from build123d import *

# Parameters (mm, degrees)
ESQUISSE1_R             = 4
BOSS_EXTRU_1_DEPTH      = 35
ESQUISSE2_R             = 3
ENL_V_MAT_EXTRU_1_DEPTH = 13
BOSS_EXTRU_2_START      = 10
BOSS_EXTRU_2_DEPTH      = 10
ESQUISSE5_R             = 10
ESQUISSE5_R_2           = 4
BOSS_EXTRU_3_DEPTH      = 7


with BuildPart() as part:
    # Esquisse1 → Boss.-Extru.1 (new body)
    with BuildSketch(Plane(origin=(0, 0, 0), x_dir=(1, 0, 0), z_dir=(0, 1, 0))):
        with Locations(Location((0, 0, 0), (0, 0, 270))):
            Circle(ESQUISSE1_R)
    extrude(amount=-BOSS_EXTRU_1_DEPTH)

    # Esquisse2 → Enlèv. mat.-Extru.1 (cut)
    with BuildSketch(Plane(origin=(0, 0, 0), x_dir=(1, 0, 0), z_dir=(0, 1, 0))):
        with Locations(Location((0, 0, 0), (0, 0, 270))):
            Circle(ESQUISSE2_R)
    extrude(amount=-ENL_V_MAT_EXTRU_1_DEPTH, mode=Mode.SUBTRACT)

    # Esquisse4 → Boss.-Extru.2 (add)
    with BuildSketch(Plane(origin=(0, -13, 0), x_dir=(1, 0, 0), z_dir=(0, 1, 0)).offset(BOSS_EXTRU_2_START)):
        with BuildLine():
            Line((-2.41, -1.786588929), (-2.41, 0))
            Line((-2.41, 0), (-2.41, 1.786588929))
            ThreePointArc((-2.41, 1.786588929), (-3, 0), (-2.41, -1.786588929))
        make_face()
    extrude(amount=-BOSS_EXTRU_2_DEPTH)

    # Esquisse5 → Boss.-Extru.3 (add)
    with BuildSketch(Plane(origin=(0, 0, 0), x_dir=(1, 0, 0), z_dir=(0, 1, 0))):
        with Locations(Location((0, 0, 0), (0, 0, 270))):
            Circle(ESQUISSE5_R)
        with Locations(Location((0, 0, 0), (0, 0, 270))):
            Circle(ESQUISSE5_R_2, mode=Mode.SUBTRACT)
    extrude(amount=-BOSS_EXTRU_3_DEPTH)


solid = part.part
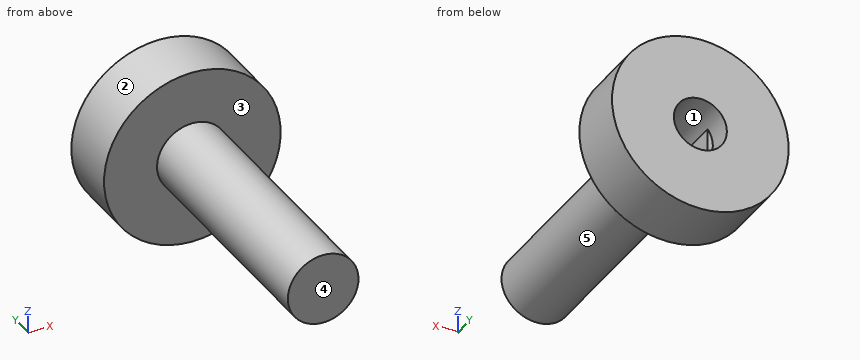
Model file for the job. Use its own axes, mm. Face numbers are marked on the shaded views. A direction names the side the tool comes from. Give positions to 0.01 mm unless a question says otherwise; leave off trailing zeros. Loops run counter-clockwise (first coordinate to the right, second up) from the corner with the lowest first, then second, coordinate; pieces in that order, holes last.
1) Wall check: line 1 (X direction, y = -10.5, z = 0); line 2 (X direction, y = -6.25, z = 0); line 3 (Y direction, x = 2.5, z = -3.75). Give the ranges that are in metal, low to high.
2) Pull direction Z, two halves, no side cores. Call the marked faces 1, 2 and 3: +Z half, -Z half, draft (parallel to the pull), parting line (faces both ways), or undercut.
3) Saw through at C-C (y = -22). Write the cut outline in (x, z).
4) Tool access for the marked faces 4 and 5: list every direction of +Z, -Z, +X, -X, +Y, -Y with a clear straight run to the whole face (end or side of a thin tool).
5) Flat gauge pins, fed straight in: pin 1 Ø6 at (y, z) = (-9.5, 5) entering from +X; pin 2 Ø5 at (x, z) = (-6.5, 1.5) entering from -Y; pin 3 Ø1.6 at (x, z) = (-0.5, 1) entering from +Y. Where does each tip first touch, or does it go through?
6) Saw through at A-A (x = 0). Write the cut outline in (y, z).
7) Saw through at D-D (y = -10.5). Write the cut outline in (x, z).
8) Saw through at B-B (z = 0). Write the cut outline in (x, y).
Answer block:
1. line 1: x = -4 to -2.41, 3 to 4
1. line 2: x = -10 to -2.41, 3 to 10
1. line 3: y = -7 to 0
2. face 1: undercut
2. face 2: parting line
2. face 3: draft
3. outline: circle Ø8 at (0, 0)
4. face 4: +Z, -Z, +X, -X, -Y
4. face 5: -Y
5. pin 1: stops at x = 9.43
5. pin 2: stops at y = -7
5. pin 3: stops at y = -13
6. outline: (-35, -4) - (-7, -4) - (-7, -10) - (0, -10) - (0, -3) - (-13, -3) - (-13, 3) - (0, 3) - (0, 10) - (-7, 10) - (-7, 4) - (-35, 4) - close
7. outline: circle Ø8 at (0, 0); hole (-2.41, -1.79) arc R3 ccw (long way) to (-2.41, 1.79) - close
8. outline: (-10, -7) - (-4, -7) - (-4, -35) - (4, -35) - (4, -7) - (10, -7) - (10, 0) - (3, 0) - (3, -13) - (-2.41, -13) - (-2.41, -3) - (-3, -3) - (-3, 0) - (-10, 0) - close
